Source: CAD feature listing. Evaluate the final solid. Frame: model axes, mm. A direction names the side the tool comes from. Round coordinates to 2 decimals unless told otherwise and drop trailing zeros. Write each loop counter-clockwise with the first axis right and the second up, starting at its lowest first coordinate (ties: lowest second). Pieces come first, ordered by that corner, then holes.
from build123d import *

# Parameters (mm, degrees)
SKETCH1_W           = 2190.75
SKETCH1_H           = 101.6
BOSS_EXTRUDE1_DEPTH = 38.1
SKETCH3_W           = 1057.275
SKETCH3_H           = 38.1
SKETCH3_W_2         = 431.8
SKETCH3_H_2         = 6.35
CUT_EXTRUDE1_DEPTH  = 19.05
SKETCH3_3_W         = 85.725
SKETCH3_3_H         = 25.4
CUT_EXTRUDE2_DEPTH  = 9.525


with BuildPart() as part:
    # Sketch1 → Boss-Extrude1 (new body)
    with BuildSketch(Plane(origin=(0, 0, 0), x_dir=(0, 0, -1), z_dir=(1, 0, 0))):
        Rectangle(SKETCH1_W, SKETCH1_H)
    extrude(amount=BOSS_EXTRUDE1_DEPTH)

    # Sketch3 → Cut-Extrude1 (cut)
    with BuildSketch(Plane.ZY):
        with Locations((-57.15, -31.75)):
            Rectangle(SKETCH3_W, SKETCH3_H)
        with Locations((879.475, -47.625)):
            Rectangle(SKETCH3_W_2, SKETCH3_H_2)
    extrude(amount=-CUT_EXTRUDE1_DEPTH, mode=Mode.SUBTRACT)

    # Sketch3_3 → Cut-Extrude2 (cut)
    with BuildSketch(Plane.ZY):
        with Locations((538.1625, -38.1)):
            Rectangle(SKETCH3_3_W, SKETCH3_3_H)
        with Locations((-652.4625, -38.1)):
            Rectangle(SKETCH3_3_W, SKETCH3_3_H)
    extrude(amount=-CUT_EXTRUDE2_DEPTH, mode=Mode.SUBTRACT)


solid = part.part
1) Section query A-A on z = -549.5. Return the cut outline in (x, y).
Taken from the geometry:
outline: (0, -12.7) - (19.05, -12.7) - (19.05, -50.8) - (38.1, -50.8) - (38.1, 50.8) - (0, 50.8) - close
2) Reachability of faces 1 (the face through (19, -1, -1095.375)), 2 (the face through (19.05, -31, -65)) from +Z, -Z, +X, -X, +Y, -Y: full face, straight path, thin tool, end or side. Return the list, or none.
Taken from the geometry:
face 1: -Z, +X, -X, +Y, -Y
face 2: -X, -Y
3) Pull-direction query (Y, two-part tool) for faces 3 (the face through (38.1, 1, 15)), 4 (the face through (19, 50.8, 15)), 5 (the face through (23, -50.8, -228)); classes: released by +Y, released by -Y, zero draft, split by the parting line, or undercut.
Taken from the geometry:
face 3: zero draft
face 4: released by +Y
face 5: released by -Y
4) Contact query for flat-ended pins moving along their axis: P1, Ø3, axis at x = 4.5, z = -643.5, coming from the -Y side; P2, Ø1.9, axis at x = 12.5, y = -48.5, coming from the +Z side (3 decimals); P3, Ø9.5, axis at x = 5.5, z = 978, coming from the -Y side. Output: stop coordinate, or through.
Taken from the geometry:
P1: stops at y = -25.4
P2: stops at z = 663.575
P3: stops at y = -44.45
5) Material intervals for line 1 (Z direction, x = 11.5, y = -45) (1 decimal); line 2 (Z direction, x = 18, y = -22.5) (1 decimal); line 3 (X direction, y = -32, z = 136.5), sorted ascending.
Taken from the geometry:
line 1: z = -1095.4 to -585.8, 471.5 to 663.6
line 2: z = -1095.4 to -585.8, 471.5 to 1095.4
line 3: x = 19.05 to 38.1
